The model under review builds one solid part; all positions refer to its coordinate system, in mm. Face numbers are marked on the shaded views. A direction names the side the tool comes from. Coordinates: 2 decimals unless noted, no trailing zeros. Loops run counter-clockwise (first coordinate to the right, second up) from the corner with the lowest first, then second, coordinate; pieces in that order, holes last. Notation, with made-up numbers: (27, 27) - (58, 27) arc R19 ccw to (58, 35) - close; hole circle Ø3 at (23.25, 69.5). An arc over 180 degrees is marked (long way). Answer in a Markdown table with one row per item. Add a question column.
(1) For line 1 along Z through (x, y) = (2.2, 3.5); line 2 along Z through (x, y) = (1.4, 3.75), list the stretches that pass through material, from the lowest coordinate up.
(2) We need section C-C on x = 3.55. Give the number of separate pieces and of enclosed holes in the cut face, plus the area to 3 significant figures.
(3) We need section B-B on z = 0. Write out the cut boundary in (x, y) (3 decimals).
(4) We need section A-A on y = 0. Write out the cut boundary in (x, z).
(5) Machinability: for the marked faces 1, 2 and 3, which of the approach directions +Z, -Z, +X, -X, +Y, -Y give a long, thin tool a straight path to every point of the face, cutting with its end or side? Answer none if there is none.
(6) For P1, Ø2, axis at x = 4, y = -3.5, coming from the -Z side; P2, Ø1.5, axis at x = 3.5, y = 1.5, coming from the +Z side; P3, Ø2, axis at x = 2, z = 4, coming from the -Y side, all flat-tipped, find the tip position at first contact; note any pin that passes through.
(7) Mouldability with a two-part tool opening along Z and no side actions: class the marked faces 4, 5 and 6 as +Z half, -Z half, draft (parallel to the pull), parting line (faces both ways), or undercut.
(8) We need section D-D on y = -2. Write out the cut boundary in (x, z) (3 decimals).
from build123d import *

# Parameters (mm, degrees)
BASPROSKE_W             = 5
BASPROSKE_H             = 5.5
TOOTHCUT_DEPTH          = 10.246621004
TEETHCUTS_COUNT         = 20
TEETHCUTS_ANGLE         = 342
BORSKE_R                = 0.5
BORE_DEPTH              = 50.0000508
SKETCH1_R               = 1.125
CUT_EXTRUDE1_DEPTH      = 10.188413972
CUT_EXTRUDE1_DEPTH_BACK = 10.188413972


with BuildPart() as part:
    # BasProSke → Base-Revolve (revolve)
    with BuildSketch(Plane(origin=(0, 0, 0), x_dir=(1, 0, 0), z_dir=(0, 1, 0)), mode=Mode.PRIVATE) as base_revolve_sk:
        with Locations((2.5, 2.75)):
            Rectangle(BASPROSKE_W, BASPROSKE_H)
    revolve(base_revolve_sk.sketch.rotate(Axis((-10, 0, 0), (1, 0, 0)), 180), axis=Axis((-10, 0, 0), (1, 0, 0)))

    # TooCutSke → ToothCut (cut, through all)
    with BuildSketch(Plane(origin=(0, 0, 0), x_dir=(0, 0, -1), z_dir=(1, 0, 0))):
        with BuildLine():
            ThreePointArc((0.249903181, 4.366855207), (0, 4.374), (-0.249903181, 4.366855207))
            ThreePointArc((-0.249903181, 4.366855207), (-0.415207844, 4.95951031), (-0.752843848, 5.473871692))
            ThreePointArc((-0.752843848, 5.473871692), (0, 5.5254), (0.752843848, 5.473871692))
            ThreePointArc((0.752843848, 5.473871692), (0.415207844, 4.95951031), (0.249903181, 4.366855207))
        make_face()
    toothcut = extrude(amount=TOOTHCUT_DEPTH, mode=Mode.SUBTRACT)

    # TeethCuts: ToothCut ×20 about axis
    teethcuts_axis = Axis((-10, 0, 0), (1, 0, 0))
    for i in range(1, TEETHCUTS_COUNT):
        add(toothcut.rotate(teethcuts_axis, i * TEETHCUTS_ANGLE / (TEETHCUTS_COUNT - 1)), mode=Mode.SUBTRACT)

    # BorSke → Bore (cut, symmetric)
    with BuildSketch(Plane(origin=(0, 0, 0), x_dir=(0, 0, -1), z_dir=(1, 0, 0))):
        with Locations(Location((0, 0, 0), (0, 0, 180))):
            Circle(BORSKE_R)
    extrude(amount=BORE_DEPTH, both=True, mode=Mode.SUBTRACT)

    # Sketch1 → Cut-Extrude1 (cut, two sides)
    with BuildSketch(Plane(origin=(5, 0, 0), x_dir=(0, 0, -1), z_dir=(1, 0, 0))) as cut_extrude1_sk:
        with Locations((0, 2)):
            Circle(SKETCH1_R)
        with Locations((0, -2)):
            Circle(SKETCH1_R)
    extrude(amount=CUT_EXTRUDE1_DEPTH, mode=Mode.SUBTRACT)
    extrude(cut_extrude1_sk.sketch, amount=-CUT_EXTRUDE1_DEPTH_BACK, mode=Mode.SUBTRACT)


solid = part.part
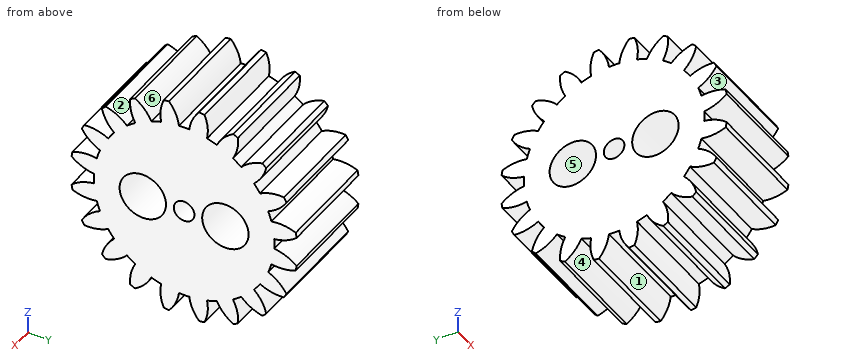
Outcome:
| question | item | result |
|---|---|---|
| 1 | line 1 | -3.89 to -2.88, -2.62 to 2.62, 2.88 to 3.89 |
| 1 | line 2 | -3.97 to -3.22, -2.4 to 2.4, 3.22 to 3.97 |
| 2 | separate pieces | 1 |
| 2 | enclosed holes | 3 |
| 2 | area | 66.9 mm² |
| 3 | outline | (0, -4.374) - (5, -4.374) - (5, -3.125) - (0, -3.125) - close; (0, -0.875) - (5, -0.875) - (5, -0.5) - (0, -0.5) - close; (0, 0.5) - (5, 0.5) - (5, 0.875) - (0, 0.875) - close; (0, 3.125) - (5, 3.125) - (5, 4.374) - (0, 4.374) - close |
| 4 | outline | (0, -4.37) - (5, -4.37) - (5, -0.5) - (0, -0.5) - close; (0, 0.5) - (5, 0.5) - (5, 4.37) - (0, 4.37) - close |
| 5 | face 1 | -Z, +X, -X |
| 5 | face 2 | +Z, +X, -X |
| 5 | face 3 | +X, -X, -Y |
| 6 | P1 | z = -4.9 |
| 6 | P2 | z = 5.45 |
| 6 | P3 | y = -3.98 |
| 7 | face 4 | -Z half |
| 7 | face 5 | undercut |
| 7 | face 6 | +Z half |
| 8 | outline | (0, -4.664) - (5, -4.664) - (5, -1.125) - (0, -1.125) - close; (0, 1.125) - (5, 1.125) - (5, 4.664) - (0, 4.664) - close |
